Verification items for the finished model (mm, model axes). A direction names the side the tool comes from. Coordinates: 2 decimals unless noted, no trailing zeros. Order: outer loops, then holes, each group sorted by start corner. A loop starts at its lowest first (then second) coordinate and runs counter-clockwise, first axis right, second up. Notation, with made-up numbers: M 88.25,84 L 145.25,84 A17 ccw 145.25,89 Z; hole C 52.5,87 d3. An arc over 180 degrees is marked long. Return JSON: item names as keys, results as strings. Group by question number.
Q1. Access from +Z, -Z, +X, -X, +Y, -Y to the whole of each face (thin tool, end or side, straight path). Record for faces 5 (the face through (2.958, 3.699, -6.715)), 6 (the face through (7.301, 14.126, 6.715)), 7 (the face through (8.3, 9.5, -7)).
Q2. Section check A-A, the plane y = 13. Enter the section's corners in (x, z).
Q3. Thickness scan on probe 1 along Y at (x, z) = (8, 0); probe 2 along X at (y, z) = (1.5, 0); probe 3 along X at (y, z) = (19.5, 3.75). Record the ranges inside material, lowest first.
Q4. Section check C-C, the plane x = 4. Enter the section's corners in (y, z).
Q5. Go/stop test with flat-tipped pins: pin 1 Ø1 at (y, z) = (21.5, 0.5) entering from -X; pin 2 Ø3.5 at (x, z) = (0.5, 1) entering from +Y; pin 3 Ø3 at (y, z) = (13, 0) entering from +X; pin 4 Ø5 at (x, y) = (5.5, 10) entering from -Z. Record where each tip stops, or that it passes through.
Q6. Section check B-B, the plane x = 1. Enter the section's corners in (y, z), then the cut area to 3 significant figures.
Q7. Mould release check, pull along Z, two halves, no side actions. Record for faces 1 (the face through (7, 17, 0)), 2 (the face through (9, 28, -4.9)), 3 (the face through (9, 15, 0)), 4 (the face through (-2, 2, 0)): pulls with the +Z half, pulls with the -Z half, needs draft (parallel to the pull), parting line crosses it, or undercut.
from build123d import *

# Parameters (mm, degrees)
SKETCH1_R           = 7
SKETCH1_R_2         = 2
BOSS_EXTRUDE1_DEPTH = 4
SKETCH2_W           = 4
SKETCH2_H           = 14
BOSS_EXTRUDE2_DEPTH = 26
CUT_EXTRUDE2_REACH  = 35.838
SKETCH4_R           = 2
FILLET6_R           = 7
FILLET7_R           = 1
FILLET8_R           = 1


with BuildPart() as part:
    # Sketch1 → Boss-Extrude1 (new body)
    # profile 1 of 2: a face of its own
    with BuildSketch(Plane(origin=(0, 0, 0), x_dir=(1, 0, 0), z_dir=(0, 1, 0))):
        Circle(SKETCH1_R)
        with Locations(Location((0, 0, 0), (0, 0, 270))):
            Circle(SKETCH1_R_2, mode=Mode.SUBTRACT)
    # profile 2 of 2: a face of its own
    with BuildSketch(Plane(origin=(0, 0, 0), x_dir=(1, 0, 0), z_dir=(0, 1, 0))):
        with BuildLine():
            Line((11, 7), (0, 7))
            ThreePointArc((0, 7), (4.949747468, 4.949747468), (7, 0))
            ThreePointArc((7, 0), (4.949747468, -4.949747468), (0, -7))
            Line((0, -7), (11, -7))
            Line((11, -7), (11, 7))
        make_face()
    extrude(amount=BOSS_EXTRUDE1_DEPTH)

    # Sketch2 → Boss-Extrude2 (add)
    with BuildSketch(Plane(origin=(0, 4, 0), x_dir=(1, 0, 0), z_dir=(0, 1, 0))):
        with Locations((9, 0)):
            Rectangle(SKETCH2_W, SKETCH2_H)
    extrude(amount=BOSS_EXTRUDE2_DEPTH)

    # Sketch4 → Cut-Extrude2 (cut, up to next)
    with BuildSketch(Plane.ZY.offset(-7), mode=Mode.PRIVATE) as cut_extrude2_sk1:
        with Locations((0, 23)):
            Circle(SKETCH4_R)
    cut_extrude2_tool1 = extrude(cut_extrude2_sk1.sketch, amount=-CUT_EXTRUDE2_REACH, mode=Mode.PRIVATE) & part.part
    # Sketch4 → Cut-Extrude2 (cut, up to next)
    with BuildSketch(Plane.ZY.offset(-7), mode=Mode.PRIVATE) as cut_extrude2_sk2:
        with Locations((0, 13)):
            Circle(SKETCH4_R)
    cut_extrude2_tool2 = extrude(cut_extrude2_sk2.sketch, amount=-CUT_EXTRUDE2_REACH, mode=Mode.PRIVATE) & part.part
    add(cut_extrude2_tool1.solids().sort_by_distance((7, 23, 0))[0], mode=Mode.SUBTRACT)
    add(cut_extrude2_tool2.solids().sort_by_distance((7, 13, 0))[0], mode=Mode.SUBTRACT)

    # Fillet6
    fillet6_edges = [part.edges().sort_by_distance(p)[0] for p in [
        (9, 30, -7),
        (9, 30, 7),
    ]]
    fillet(fillet6_edges, radius=FILLET6_R - 0.0001)  # a hair under: the kernel refuses the full size

    # Fillet7
    fillet7_edges = [part.edges().sort_by_distance(p)[0] for p in [
        (7, 4, 0),
        (11, 0, 0),
    ]]
    fillet(fillet7_edges, radius=FILLET7_R)

    # Fillet8
    fillet8_edges = [part.edges().sort_by_distance(p)[0] for p in [
        (3, 4, -7),
        (7, 14.00005, 7),
        (7, 14.00005, -7),
        (7, 27.949776758, 4.949776758),
        (7, 27.949776758, -4.949776758),
        (11, 12.00005, -7),
        (11, 12.00005, 7),
        (11, 27.949776758, 4.949776758),
        (11, 27.949776758, -4.949776758),
        (5, 0, 7),
        (3, 4, 7),
        (10.707106781, 0.292893219, 7),
        (10.707106781, 0.292893219, -7),
        (6.707106781, 4.292893219, 7),
        (6.707106781, 4.292893219, -7),
        (5, 0, -7),
        (-7, 0, 0),
        (-7, 4, 0),
    ]]
    fillet(fillet8_edges, radius=FILLET8_R)


solid = part.part
Numbers:
{
 "1": {"face 5": "-Z, -X, +Y", "face 6": "+Z, -X, +Y", "face 7": "-Z, +X, -X, +Y, -Y"},
 "2": {"outline": "M 7,-6 A1 ccw 8,-7 L 10,-7 A1 ccw 11,-6 L 11,-2 L 7,-2 Z; M 7,2 L 11,2 L 11,6 A1 ccw 10,7 L 8,7 A1 ccw 7,6 Z"},
 "3": {"probe 1": "y = 0 to 11, 15 to 21, 25 to 30", "probe 2": "x = -7 to -2, 2 to 11", "probe 3": "x = 7 to 11"},
 "4": {"outline": "M 0,-6 A1 ccw 1,-7 L 3,-7 A1 ccw 4,-6 L 4,6 A1 ccw 3,7 L 1,7 A1 ccw 0,6 Z"},
 "5": {"pin 1": "stops at x = 7", "pin 2": "stops at y = 4", "pin 3": "passes through", "pin 4": "stops at z = -7"},
 "6": {"outline": "M 0,-6 A1 ccw 1,-7 L 3,-7 A1 ccw 4,-6 L 4,-1.73 L 0,-1.73 Z; M 0,1.73 L 4,1.73 L 4,6 A1 ccw 3,7 L 1,7 A1 ccw 0,6 Z", "area": "41.3 mm2"},
 "7": {"face 1": "needs draft", "face 2": "pulls with the -Z half", "face 3": "undercut", "face 4": "undercut"}
}
